Input: dimensioned drawing with shaded views. Units: mm. Origin: part minimum x, y, z. Give positions to 0.01 mm unless a question says otherwise; leave off trailing zeros. Loops run counter-clockwise (first coordinate to the right, second up) from the corner with the lowest first, then second, coordinate; pieces in that order, holes last.
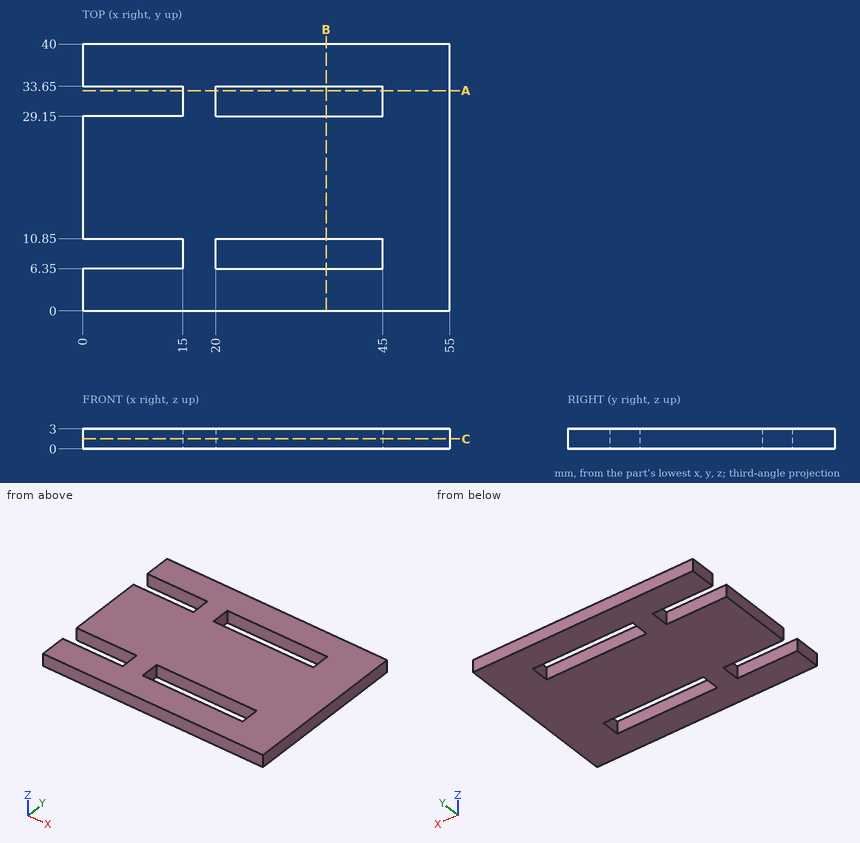
(1) First-contact query: pin 1 (0.9 mm diameter, centred on y = 31, z = 1, fed in from -X). Flat tip, straight axial feed; report the tip coordinate or a pass-through.
A:
pin 1: stops at x = 15
(2) Ray query, line 1 along Y through (x, z) = (22.5, 1.25); line 2 along X through (y, z) = (31, 0.95). Return the intervals inside material, ascending.
A:
line 1: y = 0 to 6.35, 10.85 to 29.15, 33.65 to 40
line 2: x = 15 to 20, 45 to 55
(3) Section C-C, the plane z = 1.5. Return the cut outline in (x, y).
A:
outline: (0, 0) - (55, 0) - (55, 40) - (0, 40) - (0, 33.65) - (15, 33.65) - (15, 29.15) - (0, 29.15) - (0, 10.85) - (15, 10.85) - (15, 6.35) - (0, 6.35) - close; hole (20, 6.35) - (45, 6.35) - (45, 10.85) - (20, 10.85) - close; hole (20, 29.15) - (45, 29.15) - (45, 33.65) - (20, 33.65) - close
(4) Section A-A, the plane y = 33. Return the cut outline in (x, z), then the cut area to 3 significant figures.
A:
outline: (15, 0) - (20, 0) - (20, 3) - (15, 3) - close; (45, 0) - (55, 0) - (55, 3) - (45, 3) - close
area: 45.0 mm2
(5) Section B-B, the plane x = 36.5. Return the cut outline in (y, z), then the cut area to 3 significant figures.
A:
outline: (0, 0) - (6.35, 0) - (6.35, 3) - (0, 3) - close; (10.85, 0) - (29.15, 0) - (29.15, 3) - (10.85, 3) - close; (33.65, 0) - (40, 0) - (40, 3) - (33.65, 3) - close
area: 93.0 mm2
